Verification items for the finished model (mm, model axes). A direction names the side the tool comes from. Give positions to 0.01 mm unless a question says otherwise; leave off trailing zeros. Order: outer loops, then holes, each group sorted by start corner. A loop starts at its lowest first (then second) coordinate and runs counter-clockwise, first axis right, second up. Notation, with made-up numbers: (60.25, 6) -> (115.25, 6) arc R11 ccw to (115.25, 17) -> close; hole circle Ø3 at (17.5, -35). An arc over 180 degrees is marked (long way). One line per question, with ' | ' between items. Start each with the question number.
Q1. Mould release check, pull along Y, two halves, no side actions. Record for faces 4 (the cylindrical face through (-11.172, 16.331, 12.522)), 5 (the flat face through (-11, -8, 25.4)), 6 (the cylindrical face through (1.93, 7.71, 12.52)): released by +Y, released by -Y, zero draft, split by the parting line, or undercut.
Q2. Section check D-D on x = 0. Record the cut outline in (y, z), plus the area to 3 significant figures.
Q3. Section check A-A on y = 11.43. Record the cut outline in (x, z).
Q4. Section check B-B on z = 10.75. Record the cut outline in (x, y).
Q5. Access from +Z, -Z, +X, -X, +Y, -Y to the whole of each face (thin tool, end or side, straight path). Record for faces 1 (the flat face through (0, 17.78, 13)), 2 (the flat face through (5, -46, 15.24)), 3 (the flat face through (-6, -40.64, 13)).
Q6. Go/stop test with a flat-tipped pin: pin 1 (3 mm diameter, centred on x = -5.08, y = -45.72, fed in from -Z). Record where the tip stops, or that it passes through.
Q7. Section check C-C on x = 5.08. Record the cut outline in (y, z).
Q8. Material ranges on probe 1 along Y at (x, z) = (-5.08, 18); probe 2 along X at (y, z) = (-3.5, 14.5); probe 3 along Y at (x, z) = (5.5, 14), recorded low to high. Write a range as [from, to].
from build123d import *

# Parameters (mm, degrees)
F0_R     = 4.191
F1_DEPTH = 25.4
F3_R     = 1.397
F4_DEPTH = 10.16
F2_R     = 0.762
F5_DEPTH = 5.08


with BuildPart() as f1:
    # F0 (on Top) → F1 (new body)
    with BuildSketch(Plane.XY):
        with BuildLine():
            Line((7.62, 17.78), (-7.62, 17.78))
            ThreePointArc((-7.62, 17.78), (-11.212102, 16.292102), (-12.7, 12.7))
            Line((-12.7, 12.7), (-12.7, -46.99))
            ThreePointArc((-12.7, -46.99), (-11.584077, -49.684077), (-8.89, -50.8))
            Line((-8.89, -50.8), (8.89, -50.8))
            ThreePointArc((8.89, -50.8), (11.584077, -49.684077), (12.7, -46.99))
            Line((12.7, -46.99), (12.7, 12.7))
            ThreePointArc((12.7, 12.7), (11.212102, 16.292102), (7.62, 17.78))
        make_face()
        Polygon((-10.16, -40.64), (-10.16, 0), (10.16, 0), (10.16, -40.64), (2.54, -40.64), (2.54, -46.99), (-2.54, -46.99), (-2.54, -40.64), align=None, mode=Mode.SUBTRACT)
        with Locations((0, 11.43)):
            Circle(F0_R, mode=Mode.SUBTRACT)
    extrude(amount=F1_DEPTH)

    # F3 (on face) → F4 (cut)
    with BuildSketch(Plane.XY.offset(25.4)):
        with Locations((-5.08, 5.08)):
            Circle(F3_R)
        with Locations((5.08, 5.08)):
            Circle(F3_R)
        with Locations((5.08, -45.72)):
            Circle(F3_R)
        with Locations((-5.08, -45.72)):
            Circle(F3_R)
    extrude(amount=-F4_DEPTH, mode=Mode.SUBTRACT)

    # F2 (on face) → F5 (cut)
    with BuildSketch(Plane(origin=(0, 17.78, 0), x_dir=(-1, 0, 0), z_dir=(0, 1, 0))):
        with Locations((0, 15.24)):
            Circle(F2_R)
    extrude(amount=-F5_DEPTH, mode=Mode.SUBTRACT)


solid = f1.part
Filled in:
1) face 4: released by +Y | face 5: zero draft | face 6: undercut
2) outline: (-50.8, 0) -> (-46.99, 0) -> (-46.99, 25.4) -> (-50.8, 25.4) -> close; (0, 0) -> (7.24, 0) -> (7.24, 25.4) -> (0, 25.4) -> close; (15.62, 0) -> (17.78, 0) -> (17.78, 14.48) -> (15.62, 14.48) -> close; (15.62, 16) -> (17.78, 16) -> (17.78, 25.4) -> (15.62, 25.4) -> close | area: 332 mm²
3) outline: (-12.7, 0) -> (-4.19, 0) -> (-4.19, 25.4) -> (-12.7, 25.4) -> close; (4.19, 0) -> (12.7, 0) -> (12.7, 25.4) -> (4.19, 25.4) -> close
4) outline: (-12.7, -46.99) arc R3.81 ccw to (-8.89, -50.8) -> (8.89, -50.8) arc R3.81 ccw to (12.7, -46.99) -> (12.7, 12.7) arc R5.08 ccw to (7.62, 17.78) -> (-7.62, 17.78) arc R5.08 ccw to (-12.7, 12.7) -> close; hole (-10.16, -40.64) -> (-2.54, -40.64) -> (-2.54, -46.99) -> (2.54, -46.99) -> (2.54, -40.64) -> (10.16, -40.64) -> (10.16, 0) -> (-10.16, 0) -> close; hole circle Ø8.38 at (0, 11.43)
5) face 1: +Z, -Z, +X, -X, +Y | face 2: +Z | face 3: +Z, -Z
6) pin 1: z = 0
7) outline: (-50.8, 0) -> (-40.64, 0) -> (-40.64, 25.4) -> (-44.32, 25.4) -> (-44.32, 15.24) -> (-47.12, 15.24) -> (-47.12, 25.4) -> (-50.8, 25.4) -> close; (0, 0) -> (17.78, 0) -> (17.78, 25.4) -> (6.48, 25.4) -> (6.48, 15.24) -> (3.68, 15.24) -> (3.68, 25.4) -> (0, 25.4) -> close
8) probe 1: [-50.8, -47.12], [-44.32, -40.64], [0, 3.68], [6.48, 17.78] | probe 2: [-12.7, -10.16], [10.16, 12.7] | probe 3: [-50.8, -40.64], [0, 17.78]
